Verification items for the finished model (mm, model axes). A direction names the side the tool comes from. Round coordinates to 2 decimals unless told otherwise and drop trailing zeros. Write each loop counter-clockwise with the first axis right and the second up, starting at its lowest first coordinate (ties: lowest second). Pieces come first, ordered by that corner, then holes. Notation, with made-up numbers: M 25.25,24 L 62.25,24 A24 ccw 62.25,39 Z; hole C 13.5,57 d3. An arc over 180 degrees is marked long. Write each question's results on one line, items separated by ' | '.
from build123d import *

# Parameters (mm, degrees)
ESQUISSE1_W        = 43
ESQUISSE1_H        = 22
BOSS_EXTRU_1_DEPTH = 610
BOSS_EXTRU_2_DEPTH = 15
BOSS_EXTRU_3_START = -625
BOSS_EXTRU_3_DEPTH = 15
CONG_1_R           = 4


with BuildPart() as part:
    # Esquisse1 → Boss.-Extru.1 (new body)
    with BuildSketch(Plane(origin=(0, 0, 0), x_dir=(1, 0, 0), z_dir=(0, 1, 0))):
        with Locations((21.5, 11)):
            Rectangle(ESQUISSE1_W, ESQUISSE1_H)
    extrude(amount=BOSS_EXTRU_1_DEPTH)

    # Esquisse2 → Boss.-Extru.2 (add)
    with BuildSketch(Plane(origin=(0, 610, 0), x_dir=(1, 0, 0), z_dir=(0, 1, 0))):
        with BuildLine():
            Line((11.5, 16), (31.5, 16))
            ThreePointArc((31.5, 16), (36.5, 11), (31.5, 6))
            Line((31.5, 6), (11.5, 6))
            ThreePointArc((11.5, 6), (6.5, 11), (11.5, 16))
        make_face()
    extrude(amount=BOSS_EXTRU_2_DEPTH)

    # Esquisse2<2> → Boss.-Extru.3 (add)
    with BuildSketch(Plane(origin=(0, 610, 0), x_dir=(1, 0, 0), z_dir=(0, 1, 0)).offset(BOSS_EXTRU_3_START)):
        with BuildLine():
            Line((11.5, 16), (31.5, 16))
            ThreePointArc((31.5, 16), (36.5, 11), (31.5, 6))
            Line((31.5, 6), (11.5, 6))
            ThreePointArc((11.5, 6), (6.5, 11), (11.5, 16))
        make_face()
    extrude(amount=BOSS_EXTRU_3_DEPTH)

    # Congé1
    cong_1_edges = [part.edges().sort_by_distance(p)[0] for p in [
        (0, 305, -22),
        (43, 305, -22),
        (43, 305, 0),
        (0, 305, 0),
    ]]
    fillet(cong_1_edges, radius=CONG_1_R)


solid = part.part
1) Access from +Z, -Z, +X, -X, +Y, -Y to the whole of each face (thin tool, end or side, straight path). Record for faces 1 (the flat face through (21, 617, -16)), 2 (the cylindrical face through (6.5, -7.6, -10.9)), 3 (the flat face through (21, -8, -16)), 4 (the cylindrical face through (6.5, 617.4, -10.9)), 5 (the cylindrical face through (36.5, 617.4, -11.1)).
Calculated:
face 1: -Z, +X, -X, +Y | face 2: -X, -Y | face 3: -Z, +X, -X, -Y | face 4: -X, +Y | face 5: +X, +Y
2) Sectioned sample at A-A, the plane x = 26. Record the cut outline in (y, z), and give its area (3 significant figures).
Calculated:
outline: M -15,-16 L 0,-16 L 0,-22 L 610,-22 L 610,-16 L 625,-16 L 625,-6 L 610,-6 L 610,0 L 0,0 L 0,-6 L -15,-6 Z | area: 13,700 mm²
3) Depth check by flat-ended pin: P1, Ø12, axis at x = 17.5, y = 618, coming from the +Z side; P2, Ø4.5, axis at x = 21.5, y = -11, coming from the -Z side; P3, Ø6, axis at x = 36.5, z = -19, coming from the +Y side. Enter the tip coordinate at first touch or a pass-through.
Calculated:
P1: stops at z = -6 | P2: stops at z = -16 | P3: stops at y = 610
4) Material ranges on line 1 (Y direction, x = 29.5, z = -1.5); line 2 (X direction, y = 556, z = -18.25); line 3 (X direction, y = 339, z = -19.25), recorded low to high. Write a range as [from, to].
Calculated:
line 1: y = [0, 610] | line 2: x = [0.01, 42.99] | line 3: x = [0.2, 42.8]
